Check sheet for the modelled part. Datum: model origin and axes. Units: mm. A direction names the side the tool comes from. Round coordinates to 2 decimals unless told otherwise and drop trailing zeros. Loops run counter-clockwise (first coordinate to the right, second up) from the corner with the lowest first, then second, coordinate; pieces in that order, holes last. Notation, with made-up numbers: (-13, 75) - (41, 75) arc R29 ccw to (41, 109) - close; hole circle Ø1 at (81, 54). An arc over 180 degrees is marked (long way). Put each result on its own line as item: value. Start each with the question number.
Item 1: Gauge pin test, flat ends, axial feed: pin 1 Ø12 at (y, z) = (-27, 16) entering from -X; pin 2 Ø3 at (x, y) = (19.5, -20) entering from +Z; pin 3 Ø5 at (y, z) = (-28, 2.5) entering from -X. Record the tip position at first contact, or that the pin passes through.
Item 2: Tool access check on faces 1 (the flat face through (42, -32, -3.058)), 2 (the flat face through (60.252, -15, 0)), 3 (the flat face through (42, -32, 4.75)). Record the directions out of +Z, -Z, +X, -X, +Y, -Y that give a thin tool (end or side, any length) a straight path to the whole face; none if there is none.
Item 3: Section check B-B, the plane x = 50.8. Record the cut outline in (y, z) (3 decimals).
Item 4: Section check D-D, the plane x = -8.5. Record the cut outline in (y, z).
Item 5: Section check A-A, the plane z = 0. Record the cut outline in (x, y).
Item 6: Draft check along X on faces 4 (the flat face through (20.926, -12.522, -31.172)), 5 (the cylindrical face through (56.666, -12.522, 26.143)), 6 (the flat face through (14, -38.1, -6)), 7 (the cylindrical face through (-14.274, -18.783, 0.628)). Enter one of: pulls with the +X half, pulls with the -X half, needs draft (parallel to the pull), parting line crosses it, or undercut.
Item 7: Section check C-C, the plane y = -31. Record the cut outline in (x, z) (1 decimal).
Item 8: Material ranges on line 1 along Z through (x, y) = (50.8, -17) (3 decimals); line 2 along Y through (x, z) = (30.5, 28); line 3 along Z through (x, y) = (0, -26.5), recorded low to high.
from build123d import *

# Parameters (mm, degrees)
F0_R     = 6.35
F0_R_2   = 14.2875
F1_DEPTH = 25.4
F2_DEPTH = 38.1
F3_W     = 35.03626
F3_H     = 7.807383
F4_DEPTH = 12.7


with BuildPart() as f1:
    # F0 (on Front) → F1 (new body)
    with BuildSketch(Plane.XZ):
        with BuildLine():
            ThreePointArc((-5.952169, 24.692745), (15.715834, 19.954261), (25.4, 0))
            ThreePointArc((25.4, 0), (15.715834, -19.954261), (-5.952169, -24.692745))
            Line((-5.952169, -24.692745), (48.567936, -37.83478))
            ThreePointArc((48.567936, -37.83478), (56.217416, -36.409362), (60.251547, -29.755632))
            Line((60.251547, -29.755632), (60.251547, 27.394368))
            Line((60.251547, 27.394368), (60.251547, 29.755632))
            ThreePointArc((60.251547, 29.755632), (56.217416, 36.409362), (48.567936, 37.83478))
            Line((48.567936, 37.83478), (-5.952169, 24.692745))
        make_face()
        with Locations((50.8, -28.575)):
            Circle(F0_R, mode=Mode.SUBTRACT)
        with Locations((50.8, 28.575)):
            Circle(F0_R, mode=Mode.SUBTRACT)
        with BuildLine():
            ThreePointArc((-5.952169, -24.692745), (15.715834, -19.954261), (25.4, 0))
            ThreePointArc((25.4, 0), (15.715834, 19.954261), (-5.952169, 24.692745))
            ThreePointArc((-5.952169, 24.692745), (-25.4, 0), (-5.952169, -24.692745))
        make_face()
        Circle(F0_R_2, mode=Mode.SUBTRACT)
    extrude(amount=F1_DEPTH)

    # F0 (on Front) → F2 (join)
    with BuildSketch(Plane.XZ):
        with BuildLine():
            ThreePointArc((-5.952169, -24.692745), (15.715834, -19.954261), (25.4, 0))
            ThreePointArc((25.4, 0), (15.715834, 19.954261), (-5.952169, 24.692745))
            ThreePointArc((-5.952169, 24.692745), (-25.4, 0), (-5.952169, -24.692745))
        make_face()
        Circle(F0_R_2, mode=Mode.SUBTRACT)
    extrude(amount=F2_DEPTH)

    # F3 (on face) → F4 (join)
    with BuildSketch(Plane.XZ.offset(25.4)):
        with Locations((42.733417, 0.846031)):
            Rectangle(F3_W, F3_H)
        with BuildLine():
            Line((60.251547, -3.057661), (60.251547, 4.749722))
            Line((60.251547, 4.749722), (25.215287, 4.749722))
            Line((25.215287, 4.749722), (25.215287, 3.057661))
            ThreePointArc((25.215287, 3.057661), (25.4, 0), (25.215287, -3.057661))
            Line((25.215287, -3.057661), (60.251547, -3.057661))
        make_face()
    extrude(amount=F4_DEPTH)


solid = f1.part
Check result:
1. pin 1: x = -23.35
1. pin 2: z = 31.19
1. pin 3: x = -25.4
2. face 1: -Z, +X, -Y
2. face 2: +Z, -Z, +X, +Y, -Y
2. face 3: +Z, +X, -Y
3. outline: (-38.1, -3.058) - (-25.4, -3.058) - (-25.4, -22.225) - (0, -22.225) - (0, 22.225) - (-25.4, 22.225) - (-25.4, 4.75) - (-38.1, 4.75) - close; (-25.4, -38.1) - (0, -38.1) - (0, -34.925) - (-25.4, -34.925) - close; (-25.4, 34.925) - (0, 34.925) - (0, 38.1) - (-25.4, 38.1) - close
4. outline: (-38.1, -23.94) - (0, -23.94) - (0, -11.48) - (-38.1, -11.48) - close; (-38.1, 11.48) - (0, 11.48) - (0, 23.94) - (-38.1, 23.94) - close
5. outline: (-25.4, -38.1) - (-14.29, -38.1) - (-14.29, 0) - (-25.4, 0) - close; (14.29, -38.1) - (60.25, -38.1) - (60.25, 0) - (14.29, 0) - close
6. face 4: pulls with the -X half
6. face 5: undercut
6. face 6: needs draft
6. face 7: undercut
7. outline: (-6, 24.7) arc R25.4 ccw (long way) to (25.2, -3.1) - (60.3, -3.1) - (60.3, 4.7) - (25.2, 4.7) - (25.2, 3.1) arc R25.4 ccw to start; hole circle Ø28.6 at (0, 0)
8. line 1: -38.1 to -34.925, -22.225 to 22.225, 34.925 to 38.1
8. line 2: -25.4 to 0
8. line 3: -25.4 to -14.29, 14.29 to 25.4
